Check sheet for the modelled part. Datum: model origin and axes. Units: mm. A direction names the side the tool comes from. Round coordinates to 2 decimals unless told otherwise and drop trailing zeros. Order: outer loops, then holes, each group sorted by start corner. A loop starts at its lowest first (then second) coordinate and runs counter-clockwise, first axis right, second up. Notation, with made-up numbers: (23, -21.5) -> (78, -21.5) arc R22 ccw to (78, 14.5) -> close; hole circle Ø8 at (89, 84.5). An arc over 180 degrees is marked (long way). Answer as CSV lines item,"result". Start each with the question number.
from build123d import *

# Parameters (mm, degrees)
F1_DEPTH = 310
F0_W     = 34
F0_H     = 8
F2_DEPTH = 250
F3_DEPTH = 310
F0_W_2   = 25
F4_DEPTH = 309.9
F5_R     = 13.5
F6_DEPTH = 76
F7_R     = 7.58231
F8_DEPTH = 325


with BuildPart() as f1:
    # F0 (on Front) → F1 (new body)
    with BuildSketch(Plane.XZ):
        Polygon((70.983323, 8), (52.983323, 8), (52.983323, 0), (52.983323, -19.15983), (70.983323, -19.15983), (70.983323, 3.84017), align=None)
        Polygon((-69.016677, -19.15983), (-51.016677, -19.15983), (-51.016677, 0), (-51.016677, 8), (-69.016677, 8), (-69.016677, 3.84017), align=None)
    extrude(amount=F1_DEPTH)



with BuildPart() as f2:
    # F0 (on Front) → F2 (new body)
    with BuildSketch(Plane.XZ):
        with Locations((0.983323, 4)):
            Rectangle(F0_W, F0_H)
    extrude(amount=F2_DEPTH)

    # F0 (on Front) → F3 (join)
    with BuildSketch(Plane.XZ):
        Polygon((-26.016677, 8), (-26.016677, 0), (-26.016677, -19.15983), (-16.016677, -19.15983), (-16.016677, 0), (-16.016677, 8), align=None)
        Polygon((27.983323, 8), (17.983323, 8), (17.983323, 0), (17.983323, -19.15983), (27.983323, -19.15983), (27.983323, 0), align=None)
    extrude(amount=F3_DEPTH)


with BuildPart() as f4:
    # F0 (on Front) → F4 (new body)
    with BuildSketch(Plane.XZ):
        with Locations((-38.516677, 4)):
            Rectangle(F0_W_2, F0_H)
        with Locations((40.483323, 4)):
            Rectangle(F0_W_2, F0_H)
        with Locations((0.983323, 4)):
            Rectangle(F0_W, F0_H)
    extrude(amount=F4_DEPTH)


with BuildPart() as f1_1:
    add(f1.part)

    add(f2.part)  # F6 merges F2

    add(f4.part)  # F6 merges F4
    # F5 (on Right) → F6 (join, symmetric)
    with BuildSketch(Plane.YZ):
        with Locations((-309.278336, -5.516672)):
            Circle(F5_R)
    extrude(amount=F6_DEPTH, both=True)

    # F7 (on face) → F8 (cut)
    with BuildSketch(Plane.YZ.offset(76)):
        with Locations((-309.278336, -5.516672)):
            Circle(F7_R)
    extrude(amount=-F8_DEPTH, mode=Mode.SUBTRACT)


solid = f1_1.part
1) Mould release check, pull along X, two halves, no side actions. Record for faces 1 (the face through (70.983, -153, -6)), 2 (the face through (-51.017, -153, -10)), 3 (the face through (62, -153, -19.16)): released by +X, released by -X, zero draft, split by the parting line, or undercut.
2) Access from +Z, -Z, +X, -X, +Y, -Y to the whole of each face (thin tool, end or side, straight path). Record for faces 4 (the face through (17.983, -153, -9)), 5 (the face through (-76, -303, -11)).
3) Material ranges on line 1 along X through (y, z) = (-113.5, -7.5); line 2 along Y through (x, z) = (-24, -5.5); line 3 along Z through (x, y) = (-32, -51.5), recorded low to high.
4) Depth check by flat-ended pin: pin 1 Ø10 at (y, z) = (-110, -10.5) entering from -X; pin 2 Ø5.5 at (y, z) = (-161, -12) entering from +X; pin 3 Ø4 at (x, z) = (35.5, -16) entering from -Y. Enter the tip coordinate at first touch or a pass-through.
5) Section check B-B on y = -139. Record the cut outline in (x, z), then the cut area to 3 significant figures.
Solutions:
1,face 1,"released by +X"
1,face 2,"undercut"
1,face 3,"zero draft"
2,face 4,"-Z, +Y"
2,face 5,"+Z, -Z, -X, +Y, -Y"
3,line 1,"x = -69.02 to -51.02, -26.02 to -16.02, 17.98 to 27.98, 52.98 to 70.98"
3,line 2,"y = -322.78 to -316.86, -301.7 to 0"
3,line 3,"z = 0 to 8"
4,pin 1,"stops at x = -69.02"
4,pin 2,"stops at x = 70.98"
4,pin 3,"stops at y = -319.78"
5,outline,"(-69.02, -19.16) -> (-51.02, -19.16) -> (-51.02, 0) -> (-26.02, 0) -> (-26.02, -19.16) -> (-16.02, -19.16) -> (-16.02, 0) -> (17.98, 0) -> (17.98, -19.16) -> (27.98, -19.16) -> (27.98, 0) -> (52.98, 0) -> (52.98, -19.16) -> (70.98, -19.16) -> (70.98, 8) -> (-69.02, 8) -> close"
5,area,"2,190 mm^2"
